Verification items for the finished model (mm, model axes). Face numbers are marked on the shaded views. A direction names the side the tool comes from. Give positions to 0.01 mm unless a question says otherwise; leave off trailing zeros. Write each loop counter-clockwise with the first axis right and the second up, starting at its lowest first coordinate (ties: lowest second). Pieces come first, ordered by that corner, then holes. Notation, with made-up numbers: M 52,35.5 L 98,35.5 A24 cw 98,72.5 Z; hole C 19.5,78 d2. An arc over 180 degrees is marked long. Answer as a JSON object with one key per item and string values.
Autodesk Inventor part; units mm, degrees
ref_plane "YZ Plane" through (0, 0, 0) normal (1, 0, 0) x (0, 1, 0)
ref_plane "XZ Plane" through (0, 0, 0) normal (0, 1, 0) x (-1, 0, 0)
ref_plane "XY Plane" through (0, 0, 0) normal (0, 0, 1) x (1, 0, 0)
sketch "Sketch1" plane through (0, 0, 0) normal (0, 0, 1) x (1, 0, 0)
  line L0 (-3.7, -3.65) -> (3.7, -3.65)
  line L1 (3.7, -3.65) -> (3.7, 3.65)
  line L2 (3.7, 3.65) -> (-3.7, 3.65)
  line L3 (-3.7, 3.65) -> (-3.7, -3.65)
  line L4 (-3.7, -3.65) -> (3.7, 3.65) construction
  line L5 (3.7, -3.65) -> (-3.7, 3.65) construction
  line L6 (-1.75, -3.65) -> (1.75, -3.65)
  line L7 (1.75, -3.65) -> (1.75, 0.05)
  line L8 (1.75, 0.05) -> (-1.75, 0.05)
  line L9 (-1.75, 0.05) -> (-1.75, -3.65)
  point P0 (0, 0)
  point P1 (0, 0.05)
  dimension "d0" = 7.4
  dimension "d1" = 7.3
  dimension "d2" = 3.5
  dimension "d3" = 3.7
extrude "Extrusion1" add sketch "Sketch1" along normal blind 6 contours L3 L2 L1 L0 L7 L8 L9
extrude "Extrusion2" add sketch "Sketch1" along normal blind 2 contours L9 L8 L7 L0
properties part number "Socket"
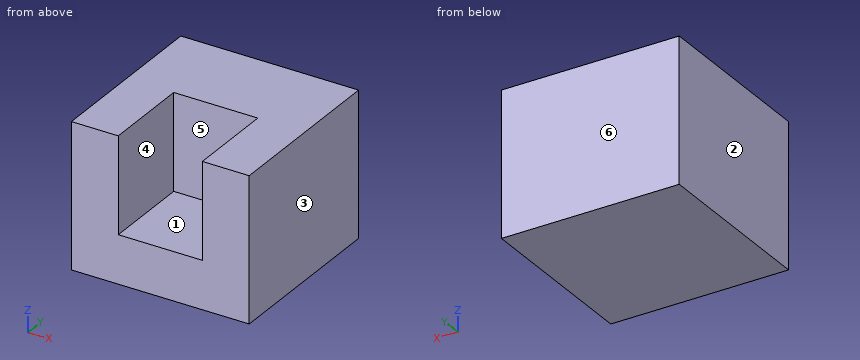
1) Go/stop test with a flat-tipped pin: pin 1 (1.8 mm diameter, centred on x = 0.5, y = -1, fed in from +Z). Record where the tip stops, or that it passes through.
Completed:
{"pin 1": "stops at z = 2"}
2) Access from +Z, -Z, +X, -X, +Y, -Y to the whole of each face (thin tool, end or side, straight path). Record for the marked faces 1 and 2.
Completed:
{"face 1": "+Z, -Y", "face 2": "+Z, -Z, -X, +Y, -Y"}
3) Release check for a two-part mould opening along X. For the marked faces 3, 4, 5 and 6 record: pulls with the +X half, pulls with the -X half, needs draft (parallel to the pull), parting line crosses it, or undercut.
Completed:
{"face 3": "pulls with the +X half", "face 4": "undercut", "face 5": "undercut", "face 6": "needs draft"}
4) Section check A-A on z = 2.7. Record the boundary of the cut face in (x, y), and give its area (3 significant figures).
Completed:
{"outline": "M -3.7,-3.65 L -1.75,-3.65 L -1.75,0.05 L 1.75,0.05 L 1.75,-3.65 L 3.7,-3.65 L 3.7,3.65 L -3.7,3.65 Z", "area": "41.1 mm2"}
5) Thickness scan on L1, parallel to X at y = -3, z = 5.75; L2, parallel to Y at x = 1.5, z = 3.7; L3, parallel to Z at x = 0.75, y = -2.75. Record the ranges inside material, lowest first.
Completed:
{"L1": "x = -3.7 to -1.75, 1.75 to 3.7", "L2": "y = 0.05 to 3.65", "L3": "z = 0 to 2"}
6) Section check B-B on y = -0.5. Record the boundary of the cut face in (x, z), and give its area (3 significant figures).
Completed:
{"outline": "M -3.7,0 L 3.7,0 L 3.7,6 L 1.75,6 L 1.75,2 L -1.75,2 L -1.75,6 L -3.7,6 Z", "area": "30.4 mm2"}
7) Section check C-C on x = -0.25. Record the boundary of the cut face in (y, z).
Completed:
{"outline": "M -3.65,0 L 3.65,0 L 3.65,6 L 0.05,6 L 0.05,2 L -3.65,2 Z"}
